from build123d import *

# Parameters (mm, degrees)
F0_W     = 127
F0_H     = 12.7
F1_DEPTH = 25.4
F2_SIZE2 = 12.69999
F2_SIZE  = 12.69999


# Not quite as in the source:
# - a fillet or chamfer is up to 0.001 mm smaller than in the source, because OpenCascade refuses the exact size


with BuildPart() as f1:
    # F0 (on Front) → F1 (new body, symmetric)
    with BuildSketch(Plane.XZ):
        with Locations((0, 6.35)):
            Rectangle(F0_W, F0_H)
    extrude(amount=F1_DEPTH, both=True)

    # F2 (size 12.7 and 12.7 in the source; OpenCascade refuses exactly that, so slightly less here)
    f2_edges = [f1.edges().sort_by_distance(p)[0] for p in [
        (63.5, 0, 12.7),
        (0, 25.4, 12.7),
        (-63.5, 0, 12.7),
        (0, -25.4, 12.7),
    ]]
    chamfer(f2_edges, length=F2_SIZE, length2=F2_SIZE2)


solid = f1.part
Here's how the part is built. I have some questions about the finished solid (model axes, mm). Coordinates: 2 decimals unless noted, no trailing zeros. Write each loop counter-clockwise with the first axis right and the second up, starting at its lowest first coordinate (ties: lowest second). Pieces come first, ordered by that corner, then holes. Notation, with made-up numbers: (9, 1.25) - (39, 1.25) arc R24 cw to (39, 33.25) - close; hole circle Ø8 at (86, 65.5). An arc over 180 degrees is marked (long way). Use one line per item in the form item = value.
1) Suppose I cut it at C-C, the plane z = 8. Write out the boundary of the cut face in (x, y), plus the area to 3 significant figures.
Solved:
outline = (-55.5, -17.4) - (55.5, -17.4) - (55.5, 17.4) - (-55.5, 17.4) - close
area = 3,860 mm2
2) I need wall thicknesses on line 1 (X direction, y = 12.5, z = 1.25); line 2 (X direction, y = 3.5, z = 6.5); line 3 (Y direction, x = 10, z = 12.25). Which ranges of each line are inside material? Lowest first, please.
Solved:
line_1 = -62.25 to 62.25
line_2 = -57 to 57
line_3 = -13.15 to 13.15
3) I'm going to push flat-ended pins straight in: P1, Ø5, axis at y = -18, z = 9, coming from the +X side; P2, Ø1.5, axis at y = -4.5, z = 6.5, coming from the +X side; P3, Ø3, axis at y = 6, z = 6.5, coming from the -X side. Where does each tip first touch, or does it pass through?
Solved:
P1 = 57
P2 = 57.75
P3 = -58.5
4) Suppose I cut it at D-D, the plane z = 2.5. Write out the boundary of the cut face in (x, y).
Solved:
outline = (-61, -22.9) - (61, -22.9) - (61, 22.9) - (-61, 22.9) - close
